Geometry: final body of the model. Coordinates: model frame, mm. A direction names the side the tool comes from. Round coordinates to 2 decimals unless told otherwise and drop trailing zeros. Order: outer loops, then holes, each group sorted by start corner. A loop starts at its lowest first (then second) coordinate and runs counter-clockwise, first axis right, second up. Notation, with made-up numbers: M 72,84 L 91,84 A18 ccw 91,101 Z; hole C 37.5,39 d4. An arc over 180 degrees is marked long. Put each result on its own line as item: value. Start each with the question number.
1) Section A-A, the plane x = 27. Return loops of the section in (y, z), then the cut area to 3 significant figures.
2) Section B-B, the plane y = 4.25. Return loops of the section in (x, z), then the cut area to 3 significant figures.
3) Draft query along X for faces 1 (the conical face through (22.63, 5.64, 8.28)), 2 (the flat face through (39.772, 3, 8)), 3 (the flat face through (16, 0, 8)). Return one class per face: pulls with the +X half, pulls with the -X half, needs draft (parallel to the pull), parting line crosses it, or undercut.
4) Section C-C, the plane x = 7. Count the separate pieces of the cut face and the enclosed holes in it, then the cut area to 3 significant figures.
5) Access query for faces 4 (the flat face through (28, 3, 10.721)), 5 (the flat face through (16, 6, 8)), 6 (the conical face through (32.91, 0.36, 8.16)). Directions: +Z, -Z, +X, -X, +Y, -Y. A direction counts if a zero-diameter tool reaches every point of the face in a straight line with its end or side. Return the directions, or none.
6) Material intervals for probe 1 along Z at (x, y) = (30, 4); probe 2 along X at (y, z) = (3, 8); probe 3 along X at (y, z) = (1.25, 7), sorted ascending. Write a range as [from, to].
7) First-contact query: P1, Ø5, axis at x = 7.77, z = 15.22, coming from the -Y side. Flat tip, straight axial feed; report the tip coordinate or a pass-through.
from build123d import *

# Parameters (mm, degrees)
CROQUIS1_W              = 47
CROQUIS1_H              = 30
CROQUIS1_R              = 3
SALIENTE_EXTRUIR1_DEPTH = 6
CHAFL_N1_SIZE           = 0.5


with BuildPart() as part:
    # Croquis1 → Saliente-Extruir1 (new body)
    with BuildSketch(Plane(origin=(0, 0, 0), x_dir=(1, 0, 0), z_dir=(0, 1, 0))):
        with Locations((16.271686308, -8.221461187)):
            Rectangle(CROQUIS1_W, CROQUIS1_H)
        with Locations(Location((7.771686308, -1.221461187, 0), (0, 0, 270))):
            Circle(CROQUIS1_R, mode=Mode.SUBTRACT)
        with Locations(Location((7.771686308, -15.221461187, 0), (0, 0, 270))):
            Circle(CROQUIS1_R, mode=Mode.SUBTRACT)
        with BuildLine():
            Line((30.271686308, -10.721461187), (25.271686308, -10.721461187))
            ThreePointArc((25.271686308, -10.721461187), (22.771686308, -8.221461187), (25.271686308, -5.721461187))
            Line((25.271686308, -5.721461187), (30.271686308, -5.721461187))
            ThreePointArc((30.271686308, -5.721461187), (32.771686308, -8.221461187), (30.271686308, -10.721461187))
        make_face(mode=Mode.SUBTRACT)
    extrude(amount=SALIENTE_EXTRUIR1_DEPTH)

    # Chaflán1
    chafl_n1_edges = [part.edges().sort_by_distance(p)[0] for p in [
        (39.771686308, 6, 8.221461187),
        (16.271686308, 6, -6.778538813),
        (32.771686308, 0, 8.221461187),
        (27.771686308, 0, 5.721461187),
        (22.771686308, 0, 8.221461187),
        (27.771686308, 0, 10.721461187),
        (32.771686308, 6, 8.221461187),
        (27.771686308, 6, 5.721461187),
        (22.771686308, 6, 8.221461187),
        (27.771686308, 6, 10.721461187),
        (7.771686308, 0, -1.778538813),
        (7.771686308, 6, -1.778538813),
        (7.771686308, 0, 12.221461187),
        (7.771686308, 6, 12.221461187),
        (-7.228313692, 6, 8.221461187),
        (16.271686308, 0, -6.778538813),
        (39.771686308, 0, 8.221461187),
        (16.271686308, 0, 23.221461187),
        (-7.228313692, 0, 8.221461187),
        (16.271686308, 6, 23.221461187),
        (-7.228313692, 3, -6.778538813),
        (39.771686308, 3, -6.778538813),
        (39.771686308, 3, 23.221461187),
        (-7.228313692, 3, 23.221461187),
    ]]
    chamfer(chafl_n1_edges, length=CHAFL_N1_SIZE)


solid = part.part
Result sheet:
1. outline: M 0,-6.28 L 0.5,-6.78 L 5.5,-6.78 L 6,-6.28 L 6,5.22 L 5.5,5.72 L 0.5,5.72 L 0,5.22 Z; M 0,11.22 L 0.5,10.72 L 5.5,10.72 L 6,11.22 L 6,22.72 L 5.5,23.22 L 0.5,23.22 L 0,22.72 Z
1. area: 149 mm2
2. outline: M -7.23,-6.28 L -6.73,-6.78 L 39.27,-6.78 L 39.77,-6.28 L 39.77,22.72 L 39.27,23.22 L -6.73,23.22 L -7.23,22.72 Z; hole C 7.77,1.22 d6; hole C 7.77,15.22 d6; hole M 25.27,5.72 L 30.27,5.72 A2.5 ccw 30.27,10.72 L 25.27,10.72 A2.5 ccw Z
2. area: 1,310 mm2
3. face 1: undercut
3. face 2: pulls with the +X half
3. face 3: needs draft
4. separate pieces: 3
4. enclosed holes: 0
4. area: 109 mm2
5. face 4: +Y, -Y
5. face 5: +Z, -Z, +X, -X, +Y
5. face 6: -Y
6. probe 1: z = [-6.78, 5.72], [10.72, 23.22]
6. probe 2: x = [-7.23, 22.78], [32.76, 39.77]
6. probe 3: x = [-7.23, 23.09], [32.45, 39.77]
7. P1: passes through
